The listing builds one solid part. Answer for the finished solid, in the listing's coordinates (mm). A direction names the side the tool comes from. Round coordinates to 2 decimals unless told otherwise and drop trailing zeros. Write each loop counter-clockwise with the first axis right and the second up, starting at its lowest first coordinate (ties: lowest second). Pieces come first, ordered by that corner, then holes.
from build123d import *

# Parameters (mm, degrees)
BOSS_EXTRUDE1_DEPTH = 15
CUT_EXTRUDE1_REACH  = 6
SKETCH2_R           = 2.75
CHAMFER1_SIZE       = 2


with BuildPart() as part:
    # Sketch1 → Boss-Extrude1 (new body)
    with BuildSketch(Plane.XY):
        Polygon((0, 0), (19, 0), (19, -4), (4, -4), (4, -30), (0, -30), align=None)
    extrude(amount=BOSS_EXTRUDE1_DEPTH)

    # Sketch2 → Cut-Extrude1 (cut, up to next)
    with BuildSketch(Plane(origin=(4, 0, 0), x_dir=(0, 0, -1), z_dir=(1, 0, 0)), mode=Mode.PRIVATE) as cut_extrude1_sk1:
        with Locations((-7.5, -20)):
            Circle(SKETCH2_R)
    cut_extrude1_tool1 = extrude(cut_extrude1_sk1.sketch, amount=-CUT_EXTRUDE1_REACH, mode=Mode.PRIVATE) & part.part
    add(cut_extrude1_tool1.solids().sort_by_distance((4, -20, 7.5))[0], mode=Mode.SUBTRACT)

    # Chamfer1
    chamfer1_edges = [part.edges().sort_by_distance(p)[0] for p in [
        (19, -2, 15),
        (19, -2, 0),
        (2, -30, 15),
        (2, -30, 0),
    ]]
    chamfer(chamfer1_edges, length=CHAMFER1_SIZE)


solid = part.part
1. For a pull along Y with two mould halves and no side action, classify faces 3 (the face through (2.028, -17.273, 7.858)), 4 (the face through (18, -2, 1)), 5 (the face through (2, -29, 1)) as released by +Y, released by -Y, zero draft, split by the parting line, or undercut.
Geometry says:
face 3: undercut
face 4: zero draft
face 5: released by -Y
2. Section B-B on y = -20 is taken. Determine the outline of the cut face in (x, z), plus the area to 3 significant figures.
Geometry says:
outline: (0, 0) - (4, 0) - (4, 4.75) - (0, 4.75) - close; (0, 10.25) - (4, 10.25) - (4, 15) - (0, 15) - close
area: 38.0 mm2
3. Straight lines are drawn through the part: line 1 along Y through (x, z) = (2.95, 7.5); line 2 along X through (y, z) = (-13.5, 9.5); line 3 along Y through (x, z) = (7, 10.5). For each, find the intervals that lie inside material, in ascending order.
Geometry says:
line 1: y = -30 to -22.75, -17.25 to 0
line 2: x = 0 to 4
line 3: y = -4 to 0
4. Given pin 1 (4.5 mm diameter, centred on x = 13.5, z = 9.5, fed in from -Y); pin 2 (8 mm diameter, centred on y = -20, z = 2.5, fed in from +X), each flat-ended and moving along its own axis, determine where each tip first touches the part or whether it passes through.
Geometry says:
pin 1: stops at y = -4
pin 2: stops at x = 4
5. Section A-A on z = 7.5 is taken. Determine the outline of the cut face in (x, y), plus the area to 3 significant figures.
Geometry says:
outline: (0, -30) - (4, -30) - (4, -22.75) - (0, -22.75) - close; (0, -17.25) - (4, -17.25) - (4, -4) - (19, -4) - (19, 0) - (0, 0) - close
area: 158 mm2
6. A tool of negligible diameter and unlimited length cuts with its end or side. For faces 1 (the face through (18, -2, 14)), 2 (the face through (4, -17, 7)), from which of +Z, -Z, +X, -X, +Y, -Y can it reach the whole face along a straight path? Write none if from no direction.
Geometry says:
face 1: +Z, +X, +Y, -Y
face 2: +Z, -Z, +X, -Y
7. Section C-C on x = 3 is taken. Determine the outline of the cut face in (y, z).
Geometry says:
outline: (-30, 2) - (-28, 0) - (0, 0) - (0, 15) - (-28, 15) - (-30, 13) - close; hole circle Ø5.5 at (-20, 7.5)
8. Section D-D on z = 14.25 is taken. Determine the outline of the cut face in (x, y).
Geometry says:
outline: (0, -28.75) - (4, -28.75) - (4, -4) - (17.75, -4) - (17.75, 0) - (0, 0) - close
